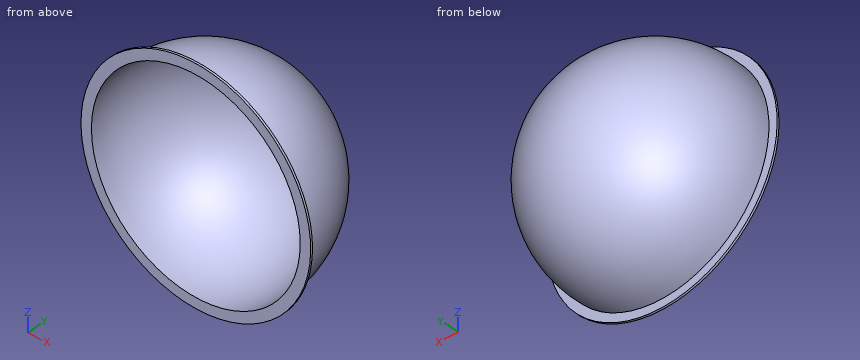
```python
from build123d import *

# Parameters (mm, degrees)
SKETCH3_R           = 177.8
BOSS_EXTRUDE1_DEPTH = 3.175


# Read off the part's stored shape, not the designer's step: Shell1
with BuildPart() as part:
    # Sketch1 → Revolve1 (revolve)
    with BuildSketch(Plane.XY):
        with BuildLine():
            Line((0, 177.8), (0, 0))
            Line((0, 0), (165.1, 0))
            ThreePointArc((165.1, 0), (121.316579658, 124.897538254), (0, 177.8))
        make_face()
    revolve(axis=Axis((0, 177.8, 0), (0, -1, 0)))

    # Sketch3 → Boss-Extrude1 (add)
    with BuildSketch(Plane.XZ):
        with Locations(Location((0, 0, 0), (0, 0, 270))):
            Circle(SKETCH3_R)
    extrude(amount=BOSS_EXTRUDE1_DEPTH)

    # Shell1 outline → Shell1 (revolve, cut)
    with BuildSketch(Plane.XY):
        with BuildLine():
            ThreePointArc((161.64461017, -3.1750001), (120.147638379, 121.477126871), (0, 174.625))
            Line((0, 174.625), (0, -3.1750001))
            Line((0, -3.1750001), (161.64461017, -3.1750001))
        make_face()
    revolve(axis=Axis((0, 0, 0), (0, 1, 0)), mode=Mode.SUBTRACT)


solid = part.part
```
Here's how the part is built. I have some questions about the finished solid (model axes, mm). Round coordinates to 2 decimals unless told otherwise and drop trailing zeros. Loops run counter-clockwise (first coordinate to the right, second up) from the corner with the lowest first, then second, coordinate; pieces in that order, holes last. Notation, with made-up numbers: (61.25, -13) -> (87.25, -13) arc R29 ccw to (87.25, 22) -> close; hole circle Ø2 at (55.5, 46). An arc over 180 degrees is marked (long way). Answer as CSV lines item,"result". Start each with the question number.
1. Imagine slicing it at B-B on x = -27. Write out the boundary of the cut face in (y, z) (3 decimals), plus the area to 3 significant figures.
2. Imagine slicing it at A-A on z = 37. Write out the boundary of the cut face in (x, y) (3 decimals).
3. I need wall thicknesses on probe 1 along X at (y, z) = (15.5, 92.5); probe 2 along X at (y, z) = (107.5, -39); probe 3 along Y at (x, z) = (-152, 83) (3 decimals). Which ranges of each line are inside material? Lowest first, please. Write a range as from..to.
4. I'm going to push flat-ended pins straight in: P1, Ø5, axis at x = 34, z = 22.5, coming from the +Y side; P2, Ø12, axis at y = 119.5, z = -32.5, coming from the -X side; P3, Ø1.5, axis at x = -4, y = 91.5, coming from the -Z side. Where does each tip first touch, or does it pass through?
5. Imagine slicing it at C-C on y = 90. Write out the boundary of the cut face in (x, z), plus the area to 3 significant figures.
Solution:
1,outline,"(-3.175, -175.738) -> (0, -175.738) -> (0, -162.877) arc R163.337 ccw (long way) to (0, 162.877) -> (0, 175.738) -> (-3.175, 175.738) -> (-3.175, 159.374) arc R160.118 cw (long way) to (-3.175, -159.374) -> close"
1,area,"1,820 mm²"
2,outline,"(-173.908, -3.175) -> (-157.353, -3.175) arc R158.107 cw (long way) to (157.353, -3.175) -> (173.908, -3.175) -> (173.908, 0) -> (160.901, 0) arc R161.366 ccw (long way) to (-160.901, 0) -> (-173.908, 0) -> close"
3,probe 1,"-137.26..-133.42, 133.42..137.26"
3,probe 2,"-129.67..-125.59, 125.59..129.67"
3,probe 3,"-3.175..0"
4,P1,"y = 173.32"
4,P2,"x = -127.11"
4,P3,"z = -145.7"
5,outline,"circle Ø292.32 at (0, 0); hole circle Ø285.1 at (0, 0)"
5,area,"3,270 mm²"
